Could you check a few things on this drawing? It's one solid part, dimensions in mm from its lowest x, y, z. Give positions to 0.01 mm unless a question says otherwise; leave off trailing zeros. Order: outer loops, then holes, each group sorted by start corner. A loop starts at its lowest first (then second) coordinate and runs counter-clockwise, first axis right, second up. Notation, with made-up numbers: (32, -5) - (73, -5) arc R25 cw to (73, 25) - close; hole circle Ø10 at (-37, -40). An arc over 180 degrees is marked (long way). Put each result on its own line as item: value.
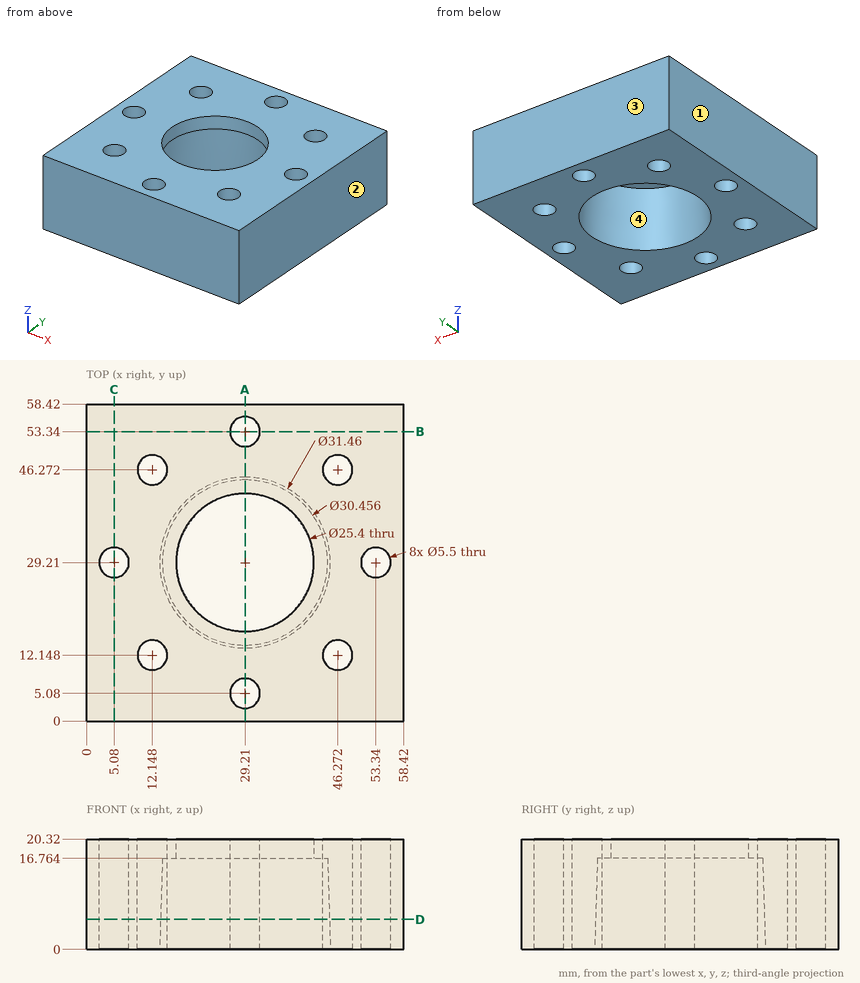
1) Suppose I cut it at D-D, the plane z = 5.5. State how many separate pieces and enclosed holes the cut face has, and give its area (3 significant figures).
Filled in:
separate pieces: 1
enclosed holes: 9
area: 2,460 mm^2
2) Suppose I cut it at A-A, the plane x = 29.21. List the corners of the cut face in (y, z) for me.
Filled in:
outline: (0, 0) - (2.33, 0) - (2.33, 20.32) - (0, 20.32) - close; (7.83, 0) - (13.48, 0) - (13.98, 16.76) - (16.51, 16.76) - (16.51, 20.32) - (7.83, 20.32) - close; (41.91, 16.76) - (44.44, 16.76) - (44.94, 0) - (50.59, 0) - (50.59, 20.32) - (41.91, 20.32) - close; (56.09, 0) - (58.42, 0) - (58.42, 20.32) - (56.09, 20.32) - close
3) I'm going to push a flat-ended pin straight in: pin 1 (7 mm diameter, centred on x = 5.08, y = 29.21, fed in from -Z). Where does the tip first touch, or does it pass through?
Filled in:
pin 1: stops at z = 0
4) Suppose I cut it at B-B, the plane y = 53.34. List the corners of the cut face in (x, z) for me, and give its area (3 significant figures).
Filled in:
outline: (0, 0) - (26.46, 0) - (26.46, 20.32) - (0, 20.32) - close; (31.96, 0) - (58.42, 0) - (58.42, 20.32) - (31.96, 20.32) - close
area: 1,080 mm^2
5) If I drill on line 1 (X direction, y = 46, z = 18.5) (1 decimal); line 2 (Y direction, x = 29.21, z = 19.5); line 3 (Y direction, x = 47, z = 17) (1 decimal), over which ranges is the centre line in solid material (lowest first)? Write a range as [from, to].
Filled in:
line 1: x = [0, 9.4], [14.9, 43.5], [49, 58.4]
line 2: y = [0, 2.33], [7.83, 16.51], [41.91, 50.59], [56.09, 58.42]
line 3: y = [0, 9.5], [14.8, 43.6], [48.9, 58.4]
6) We'd pull the mould along X, two halves only. Please class the marked faces 1, 2, 3 and 4: pulls with the +X half, pulls with the -X half, needs draft (parallel to the pull), parting line crosses it, or undercut.
Filled in:
face 1: pulls with the -X half
face 2: pulls with the +X half
face 3: needs draft
face 4: undercut
